from build123d import *

# Parameters (mm, degrees)
SKETCH1_R            = 45
BOSS_EXTRUDE1_DEPTH  = 42.5
SKETCH2_R            = 39.5
CUT_EXTRUDE1_DEPTH   = 148
DRAFT2_ANGLE         = 3
CUT_EXTRUDE2_DEPTH   = 5
SKETCH7_R            = 47.22733062
BOSS_EXTRUDE2_DEPTH  = 2
SKETCH8_R            = 39.5
CUT_EXTRUDE3_DEPTH   = 66
CUT_EXTRUDE4_DEPTH   = 15
CUT_SWEEP1_PROFILE_R = 2.25


with BuildPart() as part:
    # Sketch1 → Boss-Extrude1 (new body)
    with BuildSketch(Plane(origin=(0, 0, 0), x_dir=(1, 0, 0), z_dir=(0, 1, 0))):
        Circle(SKETCH1_R)
    extrude(amount=BOSS_EXTRUDE1_DEPTH)

    # Sketch2 → Cut-Extrude1 (cut)
    with BuildSketch(Plane(origin=(0, 42.5, 0), x_dir=(1, 0, 0), z_dir=(0, 1, 0))):
        Circle(SKETCH2_R)
    extrude(amount=-CUT_EXTRUDE1_DEPTH, mode=Mode.SUBTRACT)

    # Draft2
    draft2_faces = [part.faces().sort_by_distance(p)[0] for p in [
        (-45, 21.25, 0),
    ]]
    draft(draft2_faces, Plane.ZX.offset(42.5), DRAFT2_ANGLE)

    # Sketch6 → Cut-Extrude2 (cut)
    with BuildSketch(Plane.XZ):
        Polygon((-24.581832655, 35.879719979), (-23.131832655, 35.042562088), (-21.681832655, 37.554035759), (-18.781832655, 37.554035759), (-18.781832655, 39.22835154), (-21.681832655, 40.902667321), (-24.581832655, 39.22835154), align=None)
        Polygon((18.781832655, 39.22835154), (18.781832655, 37.554035759), (21.681832655, 37.554035759), (23.131832655, 35.042562088), (24.581832655, 35.879719979), (24.581832655, 39.22835154), (21.681832655, 40.902667321), align=None)
        Polygon((43.36366531, 0), (41.91366531, -2.511473671), (43.36366531, -3.348631561), (46.26366531, -1.674315781), (46.26366531, 1.674315781), (43.36366531, 3.348631561), (41.91366531, 2.511473671), align=None)
        Polygon((21.681832655, -37.554035759), (18.781832655, -37.554035759), (18.781832655, -39.22835154), (21.681832655, -40.902667321), (24.581832655, -39.22835154), (24.581832655, -35.879719979), (23.131832655, -35.042562088), align=None)
        Polygon((-21.681832655, -37.554035759), (-23.131832655, -35.042562088), (-24.581832655, -35.879719979), (-24.581832655, -39.22835154), (-21.681832655, -40.902667321), (-18.781832655, -39.22835154), (-18.781832655, -37.554035759), align=None)
        Polygon((-41.91366531, -2.511473671), (-43.36366531, 0), (-41.91366531, 2.511473671), (-43.36366531, 3.348631561), (-46.26366531, 1.674315781), (-46.26366531, -1.674315781), (-43.36366531, -3.348631561), align=None)
        Polygon((-41.91366531, 2.511473671), (-43.36366531, 0), (-41.91366531, -2.511473671), (-40.46366531, -1.674315781), (-40.46366531, 1.674315781), align=None)
        Polygon((-21.681832655, 37.554035759), (-23.131832655, 35.042562088), (-21.681832655, 34.205404198), (-18.781832655, 35.879719979), (-18.781832655, 37.554035759), align=None)
        Polygon((21.681832655, 37.554035759), (18.781832655, 37.554035759), (18.781832655, 35.879719979), (21.681832655, 34.205404198), (23.131832655, 35.042562088), align=None)
        Polygon((40.46366531, -1.674315781), (41.91366531, -2.511473671), (43.36366531, 0), (41.91366531, 2.511473671), (40.46366531, 1.674315781), align=None)
        Polygon((18.781832655, -35.879719979), (18.781832655, -37.554035759), (21.681832655, -37.554035759), (23.131832655, -35.042562088), (21.681832655, -34.205404198), align=None)
        Polygon((-21.681832655, -34.205404198), (-23.131832655, -35.042562088), (-21.681832655, -37.554035759), (-18.781832655, -37.554035759), (-18.781832655, -35.879719979), align=None)
    extrude(amount=-CUT_EXTRUDE2_DEPTH, mode=Mode.SUBTRACT)

    # Sketch7 → Boss-Extrude2 (add)
    with BuildSketch(Plane.XZ):
        Circle(SKETCH7_R)
    extrude(amount=-BOSS_EXTRUDE2_DEPTH)

    # Sketch8 → Cut-Extrude3 (cut)
    with BuildSketch(Plane(origin=(0, 2, 0), x_dir=(1, 0, 0), z_dir=(0, 1, 0))):
        Circle(SKETCH8_R)
    extrude(amount=-CUT_EXTRUDE3_DEPTH, mode=Mode.SUBTRACT)

    # Sketch9 → Cut-Extrude4 (cut)
    with BuildSketch(Plane.XZ):
        with BuildLine():
            Line((-42.51, 1.472243186), (-43.36, 0))
            Line((-43.36, 0), (-42.51, -1.472243186))
            ThreePointArc((-42.51, -1.472243186), (-41.887756814, -0.85), (-41.66, 0))
            ThreePointArc((-41.66, 0), (-41.887756814, 0.85), (-42.51, 1.472243186))
        make_face()
        with BuildLine():
            Line((-42.51, -1.472243186), (-43.36, 0))
            Line((-43.36, 0), (-42.51, 1.472243186))
            ThreePointArc((-42.51, 1.472243186), (-45.06, 0), (-42.51, -1.472243186))
        make_face()
        with BuildLine():
            ThreePointArc((-19.98, 37.550861508), (-22.53, 39.023104695), (-22.53, 36.078618322))
            Line((-22.53, 36.078618322), (-21.68, 37.550861508))
            Line((-21.68, 37.550861508), (-19.98, 37.550861508))
        make_face()
        with BuildLine():
            Line((-21.68, 37.550861508), (-22.53, 36.078618322))
            ThreePointArc((-22.53, 36.078618322), (-20.83, 36.078618322), (-19.98, 37.550861508))
            Line((-19.98, 37.550861508), (-21.68, 37.550861508))
        make_face()
        with BuildLine():
            ThreePointArc((23.38, 37.550861508), (21.68, 39.250861508), (19.98, 37.550861508))
            Line((19.98, 37.550861508), (21.68, 37.550861508))
            Line((21.68, 37.550861508), (22.53, 36.078618322))
            ThreePointArc((22.53, 36.078618322), (23.152243186, 36.700861508), (23.38, 37.550861508))
        make_face()
        with BuildLine():
            Line((21.68, 37.550861508), (19.98, 37.550861508))
            ThreePointArc((19.98, 37.550861508), (20.83, 36.078618322), (22.53, 36.078618322))
            Line((22.53, 36.078618322), (21.68, 37.550861508))
        make_face()
        with BuildLine():
            ThreePointArc((42.51, 1.472243186), (41.66, 0), (42.51, -1.472243186))
            Line((42.51, -1.472243186), (43.36, 0))
            Line((43.36, 0), (42.51, 1.472243186))
        make_face()
        with BuildLine():
            Line((43.36, 0), (42.51, -1.472243186))
            ThreePointArc((42.51, -1.472243186), (44.21, -1.472243186), (45.06, 0))
            ThreePointArc((45.06, 0), (44.21, 1.472243186), (42.51, 1.472243186))
            Line((42.51, 1.472243186), (43.36, 0))
        make_face()
        with BuildLine():
            ThreePointArc((22.53, -36.078618322), (20.83, -36.078618322), (19.98, -37.550861508))
            Line((19.98, -37.550861508), (21.68, -37.550861508))
            Line((21.68, -37.550861508), (22.53, -36.078618322))
        make_face()
        with BuildLine():
            Line((21.68, -37.550861508), (19.98, -37.550861508))
            ThreePointArc((19.98, -37.550861508), (21.68, -39.250861508), (23.38, -37.550861508))
            ThreePointArc((23.38, -37.550861508), (23.152243186, -36.700861508), (22.53, -36.078618322))
            Line((22.53, -36.078618322), (21.68, -37.550861508))
        make_face()
        with BuildLine():
            ThreePointArc((-19.98, -37.550861508), (-20.83, -36.078618322), (-22.53, -36.078618322))
            Line((-22.53, -36.078618322), (-21.68, -37.550861508))
            Line((-21.68, -37.550861508), (-19.98, -37.550861508))
        make_face()
        with BuildLine():
            Line((-21.68, -37.550861508), (-22.53, -36.078618322))
            ThreePointArc((-22.53, -36.078618322), (-22.53, -39.023104695), (-19.98, -37.550861508))
            Line((-19.98, -37.550861508), (-21.68, -37.550861508))
        make_face()
    extrude(amount=-CUT_EXTRUDE4_DEPTH, mode=Mode.SUBTRACT)

    # Cut-Sweep1: sweep along a path in Sketch10
    with BuildLine(Plane(origin=(0, 42.5, 0), x_dir=(1, 0, 0), z_dir=(0, 1, 0))) as cut_sweep1_path:
        CenterArc((0, 0), 42.25, 0, 360)
    # Cut-Sweep1 profile (on start of the path) → Cut-Sweep1 (sweep, cut)
    with BuildSketch(Plane(origin=(42.25, 42.5, 0), x_dir=(-1, 0, 0), z_dir=(0, 0, -1))):
        Circle(CUT_SWEEP1_PROFILE_R)
    sweep(path=cut_sweep1_path.line, mode=Mode.SUBTRACT)


solid = part.part
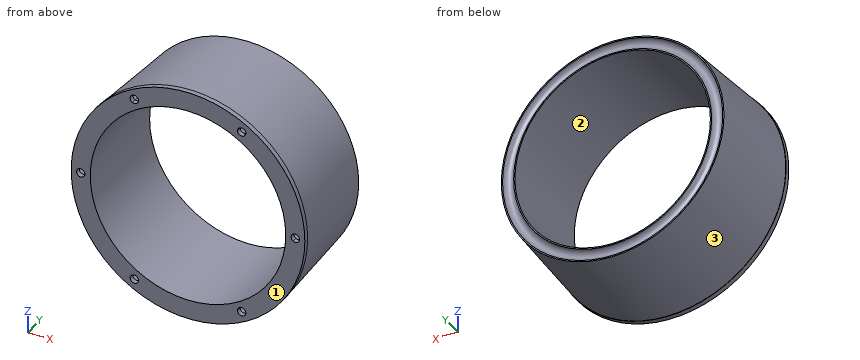
Model file for the job. Use its own axes, mm. Face numbers are marked on the shaded views. Give positions to 0.01 mm unless a question says otherwise; leave off trailing zeros. Loops run counter-clockwise (first coordinate to the right, second up) from the corner with the lowest first, then second, coordinate; pieces in that order, holes last. Notation, with made-up numbers: (40.25, -0.75) -> (48.25, -0.75) arc R31 ccw to (48.25, 26.25) -> close; hole circle Ø10 at (-36.5, 15). An arc over 180 degrees is marked (long way). Use a Markdown table: item, result. Add a question column.
(1) Wall check: line 1 along Z through (x, y) = (-21, 1); line 2 along Z through (x, y) = (23, 9.5); line 3 along X through (y, z) = (27.5, -22). Give the ranges that are in metal, low to high.
(2) Mould opens along X. For the marked faces 1, 2 and 3 say: +X half, -X half, draft (parallel to the pull), parting line (faces both ways), or undercut.
(3) Slice it at D-D on y = 16.5. List the corners of the cut face in (x, z), and give its area (3 significant figures).
(4) Slice it at A-A on x = 0. List the corners of the cut face in (y, z).
(5) Slice it at C-C on y = 32. List the corners of the cut face in (x, z), and give its area (3 significant figures).
(6) Drop flat-ended pins along their axis: pin 1 Ø4.5 at (x, z) = (-21, -36.5) entering from +Y; pin 2 Ø12 at (y, z) = (26, 24.5) entering from -X; pin 3 Ø0.9 at (y, z) = (4, 37.5) entering from -X; pin 4 Ø2.5 at (y, z) = (3, -38) entering from -X. Give the stop position or say it passes through.
(7) Slice it at B-B on y = 11.5. List the corners of the cut face in (x, z), and give its area (3 significant figures).
Filled sheet:
| question | item | result |
|---|---|---|
| 1 | line 1 | -42.3 to -39.11, -35.99 to -33.46, 33.46 to 35.99, 39.11 to 42.3 |
| 1 | line 2 | -40.68 to -38.62, -36.48 to -32.11, 32.11 to 36.48, 38.62 to 40.68 |
| 1 | line 3 | -40.15 to -32.81, 32.81 to 40.15 |
| 2 | face 1 | draft |
| 2 | face 2 | undercut |
| 2 | face 3 | parting line |
| 3 | outline | circle Ø92.73 at (0, 0); hole circle Ø79 at (0, 0) |
| 3 | area | 1,850 mm2 |
| 4 | outline | (0, -47.23) -> (2, -47.23) -> (2, -47.12) -> (42.5, -45) -> (42.5, -44.5) arc R2.25 cw to (42.5, -40) -> (42.5, -39.5) -> (0, -39.5) -> close; (0, 39.5) -> (42.5, 39.5) -> (42.5, 40) arc R2.25 cw to (42.5, 44.5) -> (42.5, 45) -> (2, 47.12) -> (2, 47.23) -> (0, 47.23) -> close |
| 5 | outline | circle Ø91.1 at (0, 0); hole circle Ø79 at (0, 0) |
| 5 | area | 1,620 mm2 |
| 6 | pin 1 | y = 42.5 |
| 6 | pin 2 | x = -41.99 |
| 6 | pin 3 | x = -28.95 |
| 6 | pin 4 | x = -29.41 |
| 7 | outline | circle Ø93.25 at (0, 0); hole circle Ø3.4 at (-43.36, 0); hole circle Ø79 at (0, 0); hole circle Ø3.4 at (-21.68, -37.55); hole circle Ø3.4 at (-21.68, 37.55); hole circle Ø3.4 at (21.68, -37.55); hole circle Ø3.4 at (21.68, 37.55); hole circle Ø3.4 at (43.36, 0) |
| 7 | area | 1,870 mm2 |
